from build123d import *

# Parameters (mm, degrees)
BOSS_EXTRUDE1_DEPTH = 3


with BuildPart() as part:
    # Sketch1 → Boss-Extrude1 (new body)
    with BuildSketch(Plane(origin=(0, 0, 0), x_dir=(0, 0, -1), z_dir=(1, 0, 0))):
        Polygon((-3, -9.935360412), (-3, -4.967680206), (-3, 0), (-20.75, -17.717680206), (-15.75, -17.717680206), (-10.75, -17.717680206), (-3, -17.717680206), align=None)
        Polygon((-3, 0), (-3, -4.967680206), (-3, -9.935360412), (0, -9.935360412), (0, 0), align=None)
        Polygon((-15.75, -17.717680206), (-20.75, -17.717680206), (-20.75, -23.717680206), (-10.75, -23.717680206), (-10.75, -17.717680206), align=None)
    extrude(amount=BOSS_EXTRUDE1_DEPTH)


solid = part.part
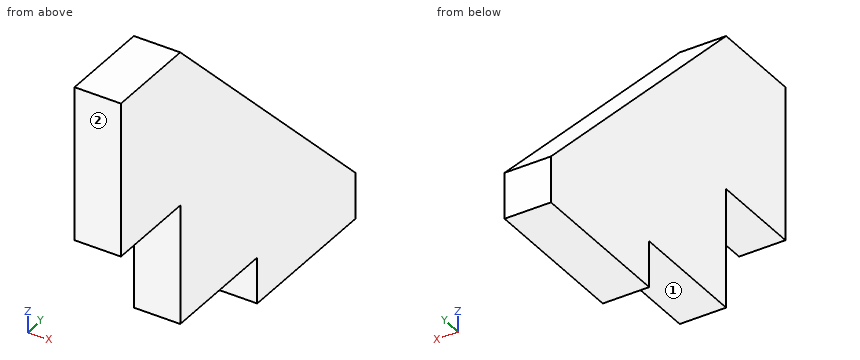
Could you check a few things on this model? Use its own coordinates, in mm. Face numbers are marked on the shaded views. A direction names the side the tool comes from. Coordinates: 2 decimals unless noted, no trailing zeros. Order: outer loops, then holes, each group sorted by start corner. A loop starts at its lowest first (then second) coordinate and runs counter-clockwise, first axis right, second up. Notation, with made-up numbers: (-4.75, 53) -> (2.25, 53) arc R16 ccw to (2.25, 79) -> close; hole circle Ø9 at (27.25, -28.75). An arc over 180 degrees is marked (long way). One line per question, with ' | ' between items.
Q1. Imagine slicing it at B-B on y = -18.25. Please give me the cut outline in (x, z), and give its area (3 significant figures).
Return value:
outline: (0, 10.75) -> (3, 10.75) -> (3, 20.75) -> (0, 20.75) -> close | area: 30.0 mm²
Q2. If I drill on L1, parallel to Z at x = 1.35, y = -20; L2, parallel to Y at x = 1.3, z = 1; L3, parallel to Z at x = 1.15, y = -1.25, over which ranges is the centre line in solid material (lowest first)?
Return value:
L1: 10.75 to 20.75 | L2: -9.94 to 0 | L3: 0 to 4.25
Q3. I'm going to push flat-ended pins straight in: P1, Ø1, axis at x = 1, z = 6, coming from the -Y side; P2, Ø0.9, axis at x = 1.5, z = 1, coming from the -Y side; P3, Ø1.5, axis at x = 1, y = -22, coming from the -Z side. Where does each tip first touch, or does it pass through?
Return value:
P1: y = -17.72 | P2: y = -9.94 | P3: z = 10.75
Q4. Imagine slicing it at A-A on x = 1. Please give me the cut outline in (y, z).
Return value:
outline: (-23.72, 10.75) -> (-17.72, 10.75) -> (-17.72, 3) -> (-9.94, 3) -> (-9.94, 0) -> (0, 0) -> (0, 3) -> (-17.72, 20.75) -> (-23.72, 20.75) -> close
Q5. On a 3-axis mill with a long thin cutter (end or side, diameter ignored), from which of +Z, -Z, +X, -X, +Y, -Y can I reach the whole of each face in a straight line? I mean the marked faces 1 and 2. Say none if no direction works.
Return value:
face 1: -Z, +X, -X, -Y | face 2: +Z, -Z, +X, -X, -Y
Q6. Imagine slicing it at C-C on z = 7.25. Please give me the cut outline in (x, y), and give its area (3 significant figures).
Return value:
outline: (0, -17.72) -> (3, -17.72) -> (3, -4.24) -> (0, -4.24) -> close | area: 40.4 mm²
